CAD build for the part. Positions are in the model's coordinates, mm. Coordinates: 2 decimals unless noted, no trailing zeros. Loops run counter-clockwise (first coordinate to the right, second up) from the corner with the lowest first, then second, coordinate; pieces in that order, holes last.
1) Pin check, flat tip, straight feed: pin 1 Ø1.5 at (x, y) = (2.5, 1.5) entering from -Z. Stop position of the tip, or through.
2) Wall check: line 1 along Y through (x, z) = (-8, 1); line 2 along Y through (x, z) = (-13, 1); line 3 along X through (y, z) = (3.5, 0.7). Give the ranges that are in metal, low to high.
3) Saw through at A-A, the plane x = -8. Write the cut outline in (y, z).
4) Saw through at C-C, the plane z = 0.9. Write the cut outline in (x, y).
5) Saw through at B-B, the plane y = 0. Write the cut outline in (x, z), and give its area (3 significant figures).
6) Saw through at D-D, the plane x = 13. Write the cut outline in (y, z).
Autodesk Inventor part; units mm, degrees
ref_plane "YZ Plane" through (0, 0, 0) normal (1, 0, 0) x (0, 1, 0)
ref_plane "XZ Plane" through (0, 0, 0) normal (0, 1, 0) x (-1, 0, 0)
ref_plane "XY Plane" through (0, 0, 0) normal (0, 0, 1) x (1, 0, 0)
sketch "スケッチ1" plane through (0, 0, 0) normal (0, 0, 1) x (1, 0, 0)
  line L0 (16, -4) -> (-16, -4)
  line L1 (-16, -4) -> (-16, 4)
  line L2 (-16, 4) -> (16, 4)
  line L3 (16, 4) -> (16, -4)
  line L4 (16, -4) -> (-16, 4) construction
  line L5 (-16, -4) -> (16, 4) construction
  circle A0 centre (8, 0) radius 0.75
  circle A1 centre (13, 0) radius 1.05
  circle A2 centre (-8, 0) radius 0.75
  circle A3 centre (-13, 0) radius 1.05
  point P0 (0, 0)
  point P1 (0, 0)
  point P2 (0, 0)
  dimension "d0" = 8
  dimension "d1" = 8
  dimension "d2" = 8
  dimension "d3" = 1.5
  dimension "d4" = 2.1
  dimension "d5" = 13
  dimension "d6" = 3
  dimension "d7" = 13
extrude "押し出し1" add sketch "スケッチ1" along normal blind 1.6
fillet "フィレット1" radius 2 4 edges at (-16, 4, 0.8) (16, 4, 0.8) (16, -4, 0.8) (-16, -4, 0.8)
properties part number "Parts_PCB_BatteryProbePCB" material "ガラス繊維バット"
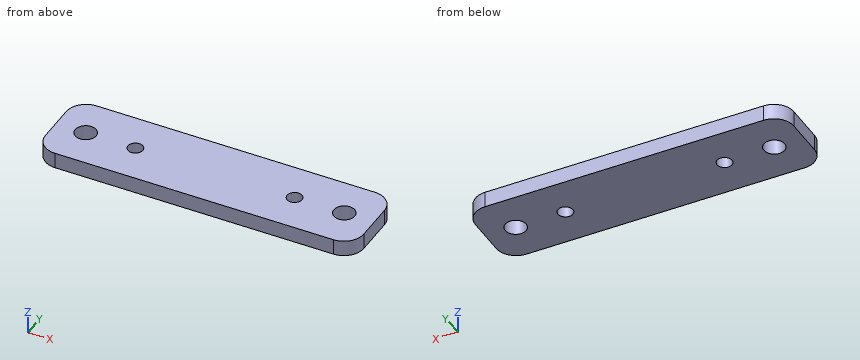
Data:
1. pin 1: stops at z = 0
2. line 1: y = -4 to -0.75, 0.75 to 4
2. line 2: y = -4 to -1.05, 1.05 to 4
2. line 3: x = -15.32 to 15.32
3. outline: (-4, 0) - (-0.75, 0) - (-0.75, 1.6) - (-4, 1.6) - close; (0.75, 0) - (4, 0) - (4, 1.6) - (0.75, 1.6) - close
4. outline: (-16, -2) arc R2 ccw to (-14, -4) - (14, -4) arc R2 ccw to (16, -2) - (16, 2) arc R2 ccw to (14, 4) - (-14, 4) arc R2 ccw to (-16, 2) - close; hole circle Ø2.1 at (-13, 0); hole circle Ø1.5 at (-8, 0); hole circle Ø1.5 at (8, 0); hole circle Ø2.1 at (13, 0)
5. outline: (-16, 0) - (-14.05, 0) - (-14.05, 1.6) - (-16, 1.6) - close; (-11.95, 0) - (-8.75, 0) - (-8.75, 1.6) - (-11.95, 1.6) - close; (-7.25, 0) - (7.25, 0) - (7.25, 1.6) - (-7.25, 1.6) - close; (8.75, 0) - (11.95, 0) - (11.95, 1.6) - (8.75, 1.6) - close; (14.05, 0) - (16, 0) - (16, 1.6) - (14.05, 1.6) - close
5. area: 39.7 mm2
6. outline: (-4, 0) - (-1.05, 0) - (-1.05, 1.6) - (-4, 1.6) - close; (1.05, 0) - (4, 0) - (4, 1.6) - (1.05, 1.6) - close
